from build123d import *

# Parameters (mm, degrees)
SKETCH1_W            = 406.4
SKETCH1_H            = 233.426
SKETCH1_W_2          = 25.4
SKETCH1_H_2          = 25.4
BOSS_EXTRUDE1_DEPTH  = 25.4
LPATTERN2_COUNT      = 2
LPATTERN2_PITCH      = 238.572
SKETCH2_W            = 25.4
SKETCH2_H            = 25.4
BOSS_EXTRUDE2_DEPTH  = 213.172
LPATTERN4_COUNT      = 2
LPATTERN4_PITCH      = 426.4
LPATTERN4_COUNT_DIR2 = 2
LPATTERN4_PITCH_DIR2 = 258.572


with BuildPart() as part:
    # Sketch1 → Boss-Extrude1 (new body)
    # profile 1 of 2: a face of its own
    with BuildSketch(Plane(origin=(0, 0, 0), x_dir=(1, 0, 0), z_dir=(0, 1, 0))):
        Polygon((-203.2, 142.113), (-203.2, 116.713), (-228.6, 116.713), (-228.6, -142.113), (228.6, -142.113), (228.6, 142.113), align=None)
        Rectangle(SKETCH1_W, SKETCH1_H, mode=Mode.SUBTRACT)
    # profile 2 of 2: a face of its own
    with BuildSketch(Plane(origin=(0, 0, 0), x_dir=(1, 0, 0), z_dir=(0, 1, 0))):
        with Locations((-215.9, 129.413)):
            Rectangle(SKETCH1_W_2, SKETCH1_H_2)
    extrude(amount=BOSS_EXTRUDE1_DEPTH)


with BuildPart() as lpattern2_1:
    # LPattern2: pattern copy
    add(part.part.moved(Location(Vector(0, 1, 0) * (1 * LPATTERN2_PITCH))))


with BuildPart() as part_1:
    add(part.part)

    add(lpattern2_1.part)  # Boss-Extrude2 merges LPattern2_1
    # Sketch2 → Boss-Extrude2 (add)
    with BuildSketch(Plane(origin=(0, 25.4, 0), x_dir=(1, 0, 0), z_dir=(0, 1, 0))):
        with Locations((-215.9, 129.413)):
            Rectangle(SKETCH2_W, SKETCH2_H)
    boss_extrude2 = extrude(amount=BOSS_EXTRUDE2_DEPTH)

    # LPattern4: Boss-Extrude2 2 × 2
    with Locations(*[(i * LPATTERN4_PITCH, 0, j * LPATTERN4_PITCH_DIR2) for i in range(LPATTERN4_COUNT) for j in range(LPATTERN4_COUNT_DIR2) if (i, j) != (0, 0)]):
        add(boss_extrude2)


solid = part_1.part
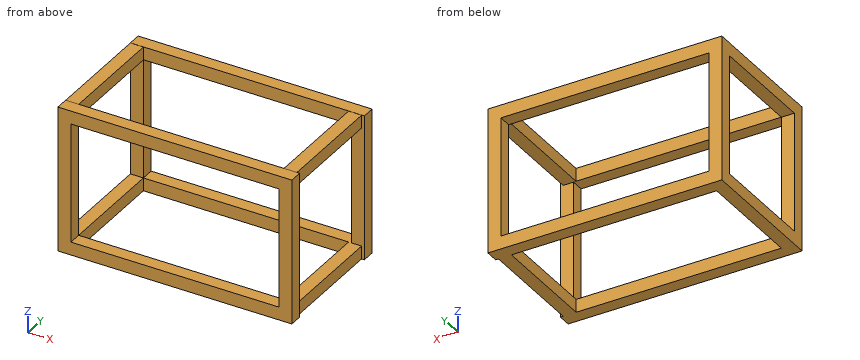
Could you check a few things on this model? Use its own coordinates, in mm. Coordinates: 2 decimals unless noted, no trailing zeros. Order: outer loops, then holes, each group sorted by start corner. A loop starts at its lowest first (then second) coordinate and runs counter-clockwise, first axis right, second up.
Q1. Will this pin go through, and if not, where does the flat tip stop? pin 1 (12.5 mm diameter, centred on y = 119, z = -133.5, fed in from +X).
Q2. Suppose I cut it at A-A on z = -23. Please give me the cut outline in (x, y), and give its area (3 significant figures).
Q3. Suppose I cut it at C-C on y = 17.5. Please give me the cut outline in (x, z).
Q4. Suppose I cut it at B-B on x = -183. Please give me the cut outline in (y, z).
Q5. Please list where these lines run through material, in increasing order: L1, parallel to Z at x = 50.5, y = 244.5; L2, parallel to Y at x = 209, z = -105.5; L3, parallel to X at y = 174, z = 125.
Answer:
1. pin 1: stops at x = 223.2
2. outline: (-228.6, 0) - (-203.2, 0) - (-203.2, 25.4) - (-228.6, 25.4) - close; (-228.6, 238.57) - (-203.2, 238.57) - (-203.2, 263.97) - (-228.6, 263.97) - close; (203.2, 0) - (228.6, 0) - (228.6, 25.4) - (203.2, 25.4) - close; (203.2, 238.57) - (228.6, 238.57) - (228.6, 263.97) - (203.2, 263.97) - close
2. area: 2,580 mm2
3. outline: (-228.6, -142.11) - (228.6, -142.11) - (228.6, 142.11) - (-228.6, 142.11) - close; hole (-203.2, -116.71) - (203.2, -116.71) - (203.2, 116.71) - (-203.2, 116.71) - close
4. outline: (0, -142.11) - (25.4, -142.11) - (25.4, -116.71) - (0, -116.71) - close; (0, 116.71) - (25.4, 116.71) - (25.4, 142.11) - (0, 142.11) - close; (238.57, -142.11) - (263.97, -142.11) - (263.97, -116.71) - (238.57, -116.71) - close; (238.57, 116.71) - (263.97, 116.71) - (263.97, 142.11) - (238.57, 142.11) - close
5. L1: z = -142.11 to -116.71, 116.71 to 142.11
5. L2: y = 0 to 25.4, 238.57 to 263.97
5. L3: x = -228.6 to -203.2, 197.8 to 223.2
